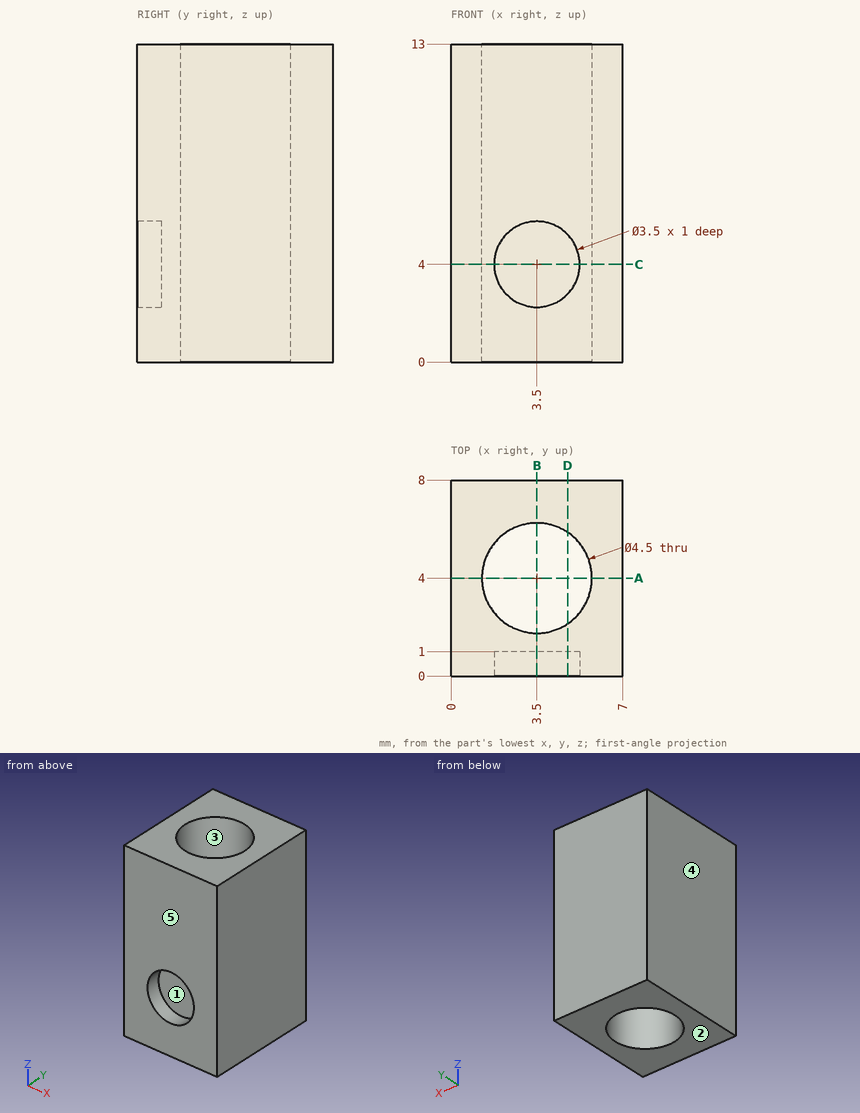
Study the drawing (mm; zero at the part's minimum x, y, z) and answer. A direction names the side the tool comes from. Coordinates: 2 decimals unless noted, no trailing zeros. Write each loop counter-clockwise with the first axis right and the second up, starting at its lowest first coordinate (ties: lowest second). Pieces come first, ordered by that corner, then holes. Notation, with made-up numbers: M 67,-27.5 L 94,-27.5 A30 ccw 94,6.5 Z; hole C 70.5,72 d6. An arc over 180 degrees is marked long. Use one line per item in the form item = value.
Item 1: Find section A-A, the plane y = 4. Give the vertices of the cut face in (x, z).
Model answer:
outline = M 0,0 L 1.25,0 L 1.25,13 L 0,13 Z; M 5.75,0 L 7,0 L 7,13 L 5.75,13 Z
Item 2: The mould has two halves that part along X. Classify the marked faces 3, 4 and 5: released by +X, released by -X, zero draft, split by the parting line, or undercut.
Model answer:
face_3 = undercut
face_4 = released by -X
face_5 = zero draft
Item 3: Given P1, Ø1.8, axis at x = 4, z = 4, coming from the -Y side, flat-ended and moving along its own axis, determine where the tip first touches the part or whether it passes through.
Model answer:
P1 = 1
Item 4: Find section B-B, the plane x = 3.5. Give the vertices of the cut face in (y, z), plus the area to 3 significant figures.
Model answer:
outline = M 0,0 L 1.75,0 L 1.75,13 L 0,13 L 0,5.75 L 1,5.75 L 1,2.25 L 0,2.25 Z; M 6.25,0 L 8,0 L 8,13 L 6.25,13 Z
area = 42.0 mm2
Item 5: Find section D-D, the plane x = 4.75. Give the vertices of the cut face in (y, z), plus the area to 3 significant figures.
Model answer:
outline = M 0,0 L 2.13,0 L 2.13,13 L 0,13 L 0,5.22 L 1,5.22 L 1,2.78 L 0,2.78 Z; M 5.87,0 L 8,0 L 8,13 L 5.87,13 Z
area = 52.9 mm2
Item 6: For the marked faces 1 and 2, determine the directions among +Z, -Z, +X, -X, +Y, -Y from which every point of the face is accessible in a straight line to the end or side of a thin tool.
Model answer:
face_1 = -Y
face_2 = -Z, +X, -X, +Y, -Y
Item 7: Find the intervals of material crossed by probe 1 along X at (y, z) = (4, 4); probe 2 along Y at (x, z) = (3.5, 4.75); probe 3 along X at (y, z) = (0.5, 4), in increasing order.
Model answer:
probe_1 = 0 to 1.25, 5.75 to 7
probe_2 = 1 to 1.75, 6.25 to 8
probe_3 = 0 to 1.75, 5.25 to 7
Item 8: Find section C-C, the plane z = 4. Give the vertices of the cut face in (x, y).
Model answer:
outline = M 0,0 L 1.75,0 L 1.75,1 L 5.25,1 L 5.25,0 L 7,0 L 7,8 L 0,8 Z; hole C 3.5,4 d4.5
